Autodesk Inventor part; units mm, degrees
ref_plane "YZ Plane" through (0, 0, 0) normal (1, 0, 0) x (0, 1, 0)
ref_plane "XZ Plane" through (0, 0, 0) normal (0, 1, 0) x (-1, 0, 0)
ref_plane "XY Plane" through (0, 0, 0) normal (0, 0, 1) x (1, 0, 0)
sketch "Sketch1" plane through (0, 0, 0) normal (0, 1, 0) x (-1, 0, 0)
  circle A0 centre (0, 0) radius 25
  dimension "d1" = 50
extrude "Extrusion1" add sketch "Sketch1" along normal blind 12
sketch "Sketch2" plane through (0, 12, 0) normal (0, 1, 0) x (1, 0, 0)
  circle A0 centre (0, 0) radius 1.3723
  line L0 (-24.9867, -1.3423) -> (-24.9867, 1.3423) construction
  line L1 (-24.2459, -0.6015) -> (-24.2459, 0.6015)
  line L2 (-25.7274, 0.6015) -> (-25.7274, -0.6015)
  arc A1 (-25.7274, -0.6015) -> (-24.2459, -0.6015) centre (-24.9867, -0.6015) ccw
  arc A2 (-24.2459, 0.6015) -> (-25.7274, 0.6015) centre (-24.9867, 0.6015) ccw
  line L3 (1.3423, -24.9867) -> (-1.3423, -24.9867) construction
  line L4 (0.6015, -24.2459) -> (-0.6015, -24.2459)
  line L5 (-0.6015, -25.7274) -> (0.6015, -25.7274)
  arc A3 (0.6015, -25.7274) -> (0.6015, -24.2459) centre (0.6015, -24.9867) ccw
  arc A4 (-0.6015, -24.2459) -> (-0.6015, -25.7274) centre (-0.6015, -24.9867) ccw
  line L6 (24.9867, 1.3423) -> (24.9867, -1.3423) construction
  line L7 (24.2459, 0.6015) -> (24.2459, -0.6015)
  line L8 (25.7274, -0.6015) -> (25.7274, 0.6015)
  arc A5 (25.7274, 0.6015) -> (24.2459, 0.6015) centre (24.9867, 0.6015) ccw
  arc A6 (24.2459, -0.6015) -> (25.7274, -0.6015) centre (24.9867, -0.6015) ccw
  line L9 (-1.3423, 24.9867) -> (1.3423, 24.9867) construction
  line L10 (-0.6015, 24.2459) -> (0.6015, 24.2459)
  line L11 (0.6015, 25.7274) -> (-0.6015, 25.7274)
  arc A7 (-0.6015, 25.7274) -> (-0.6015, 24.2459) centre (-0.6015, 24.9867) ccw
  arc A8 (0.6015, 24.2459) -> (0.6015, 25.7274) centre (0.6015, 24.9867) ccw
  point P0 (-24.9867, 0)
  point P1 (0, -24.9867)
  point P2 (24.9867, 0)
  point P3 (0, 24.9867)
  dimension "d11" = 360
extrude "Extrusion2" cut sketch "Sketch2" against normal blind 12 contours A1 L2 A2 L1 | A3 L5 A4 L4 | A5 L8 A6 L7 | A7 L11 A8 L10
sketch "Sketch3" plane through (0, 12, 0) normal (0, 1, 0) x (1, 0, 0)
  circle A0 centre (0, 0) radius 22.8086
  arc A1 (13.2024, 18.5991) -> (2.9253, 22.6202) centre (0, 0) ccw construction
  arc A2 (13.9039, 19.5873) -> (3.0807, 23.822) centre (0, 0) ccw
  arc A3 (12.501, 17.611) -> (2.7699, 21.4184) centre (0, 0) ccw
  arc A4 (12.501, 17.611) -> (13.9039, 19.5873) centre (13.2024, 18.5991) ccw
  arc A5 (3.0807, 23.822) -> (2.7699, 21.4184) centre (2.9253, 22.6202) ccw
  line L0 (0, 0) -> (13.2024, 18.5991) construction
  line L1 (0, 0) -> (2.9253, 22.6202) construction
  arc A6 (-4.0188, 23.6818) -> (-14.6663, 19.0231) centre (0, 0) ccw
  arc A7 (-14.6663, 19.0231) -> (-13.1865, 17.1037) centre (-13.9264, 18.0634) ccw
  arc A8 (-3.6133, 21.2924) -> (-13.1865, 17.1037) centre (0, 0) ccw
  arc A9 (-3.6133, 21.2924) -> (-4.0188, 23.6818) centre (-3.816, 22.4871) ccw
  arc A10 (-19.5873, 13.9039) -> (-23.822, 3.0807) centre (0, 0) ccw
  arc A11 (-23.822, 3.0807) -> (-21.4184, 2.7699) centre (-22.6202, 2.9253) ccw
  arc A12 (-17.611, 12.501) -> (-21.4184, 2.7699) centre (0, 0) ccw
  arc A13 (-17.611, 12.501) -> (-19.5873, 13.9039) centre (-18.5991, 13.2024) ccw
  arc A14 (-23.6818, -4.0188) -> (-19.0231, -14.6663) centre (0, 0) ccw
  arc A15 (-19.0231, -14.6663) -> (-17.1037, -13.1865) centre (-18.0634, -13.9264) ccw
  arc A16 (-21.2924, -3.6133) -> (-17.1037, -13.1865) centre (0, 0) ccw
  arc A17 (-21.2924, -3.6133) -> (-23.6818, -4.0188) centre (-22.4871, -3.816) ccw
  arc A18 (-13.9039, -19.5873) -> (-3.0807, -23.822) centre (0, 0) ccw
  arc A19 (-3.0807, -23.822) -> (-2.7699, -21.4184) centre (-2.9253, -22.6202) ccw
  arc A20 (-12.501, -17.611) -> (-2.7699, -21.4184) centre (0, 0) ccw
  arc A21 (-12.501, -17.611) -> (-13.9039, -19.5873) centre (-13.2024, -18.5991) ccw
  arc A22 (4.0188, -23.6818) -> (14.6663, -19.0231) centre (0, 0) ccw
  arc A23 (14.6663, -19.0231) -> (13.1865, -17.1037) centre (13.9264, -18.0634) ccw
  arc A24 (3.6133, -21.2924) -> (13.1865, -17.1037) centre (0, 0) ccw
  arc A25 (3.6133, -21.2924) -> (4.0188, -23.6818) centre (3.816, -22.4871) ccw
  arc A26 (19.5873, -13.9039) -> (23.822, -3.0807) centre (0, 0) ccw
  arc A27 (23.822, -3.0807) -> (21.4184, -2.7699) centre (22.6202, -2.9253) ccw
  arc A28 (17.611, -12.501) -> (21.4184, -2.7699) centre (0, 0) ccw
  arc A29 (17.611, -12.501) -> (19.5873, -13.9039) centre (18.5991, -13.2024) ccw
  arc A30 (23.6818, 4.0188) -> (19.0231, 14.6663) centre (0, 0) ccw
  arc A31 (19.0231, 14.6663) -> (17.1037, 13.1865) centre (18.0634, 13.9264) ccw
  arc A32 (21.2924, 3.6133) -> (17.1037, 13.1865) centre (0, 0) ccw
  arc A33 (21.2924, 3.6133) -> (23.6818, 4.0188) centre (22.4871, 3.816) ccw
  dimension "d15" = 28
  dimension "d18" = 360
extrude "Extrusion3" cut sketch "Sketch3" against normal blind 12 contours A33 A32 A31 A0 | A0 A31 A30 A33 | A27 A26 A29 A0 | A0 A29 A28 A27 | A4 A3 A5 A0 | A0 A5 A2 A4 | A23 A22 A25 A0 | A0 A25 A24 A23 | A9 A8 A7 A0 | A0 A7 A6 A9 | A19 A18 A21 A0 | A0 A21 A20 A19 | A13 A12 A11 A0 | A0 A11 A10 A13 | A15 A14 A17 A0 | A0 A17 A16 A15
sketch "Sketch4" plane through (0, 12, 0) normal (0, 1, 0) x (1, 0, 0)
  circle A0 centre (0, 0) radius 4.43
  dimension "d22" = 8.86
extrude "Extrusion4" cut sketch "Sketch4" against normal blind 12
thread "Thread1"
sketch "Sketch5" plane through (0, 12, 0) normal (0, 1, 0) x (1, 0, 0)
  circle A0 centre (0, 0) radius 4.43
extrude "Extrusion5" [suppressed]
thread "Thread3"
thread "Thread4"
properties part number "ICRC wrist model"
Here's how the part is built. I have some questions about the finished solid (model axes, mm). A direction names the side the tool comes from. Coordinates: 2 decimals unless noted, no trailing zeros. Order: outer loops, then holes, each group sorted by start corner. A loop starts at its lowest first (then second) coordinate and runs counter-clockwise, first axis right, second up.
1) Imagine slicing it at C-C on z = -9. List the corners of the cut face in (x, y) for me, and give its area (3 significant figures).
2) I need wall thicknesses on line 1 (X direction, y = 6.75, z = 6); line 2 (Z direction, x = 18, y = 10); line 3 (Z direction, x = 5, y = 1.5). Which ranges of each line are inside material? Lowest first, please.
3) Imagine slicing it at B-B on x = 0. List the corners of the cut face in (y, z) for me, and give its area (3 significant figures).
4) We'd pull the mould along X, two halves only. Please class faces 1 (the face through (24.246, 6, 0)), 2 (the face through (22.04, 6.08, -9.55)): +X half, -X half, draft (parallel to the pull), parting line (faces both ways), or undercut.
5) Imagine slicing it at D-D on x = -7.5. List the corners of the cut face in (y, z) for me.
6) Imagine slicing it at A-A on z = 0. List the corners of the cut face in (x, y) for me.
7) Which directions (+Z, -Z, +X, -X, +Y, -Y) give clear straight access to the entire face, cutting with the end or side of a thin tool? Please do faces 3 (the face through (8.83, 6.08, -22.34)), 4 (the face through (17.496, 5.916, -17.858)).
8) Will these pins go through, and if not, where does the flat tip stop? pin 1 (4 mm diameter, centred on x = 5.5, y = 5, fed in from +Z); pin 2 (4 mm diameter, centred on y = 3.5, z = 18.5, fed in from +X); pin 3 (12 mm diameter, centred on x = -0.5, z = -3, fed in from -Y); pin 4 (1.3 mm diameter, centred on y = 8, z = 0, fed in from -X).
Response values:
1. outline: (-23.32, 0) - (-22.27, 0) - (-22.27, 12) - (-23.32, 12) - close; (-19.63, 0) - (19.63, 0) - (19.63, 12) - (-19.63, 12) - close; (22.27, 0) - (23.32, 0) - (23.32, 12) - (22.27, 12) - close
1. area: 496 mm2
2. line 1: x = -24.27 to -23.26, -20.75 to 20.75, 23.26 to 24.27
2. line 2: z = -17.35 to -15.14, -11.93 to 11.93, 14.26 to 17.35
2. line 3: z = -24.49 to -23.49, -21.01 to 21.01, 23.49 to 24.49
3. outline: (0, -24.25) - (12, -24.25) - (12, -4.43) - (0, -4.43) - close; (0, 4.43) - (12, 4.43) - (12, 24.25) - (0, 24.25) - close
3. area: 476 mm2
4. face 1: +X half
4. face 2: undercut
5. outline: (0, -23.85) - (12, -23.85) - (12, -22.82) - (0, -22.82) - close; (0, -20.25) - (12, -20.25) - (12, 20.25) - (0, 20.25) - close; (0, 22.82) - (12, 22.82) - (12, 23.85) - (0, 23.85) - close
6. outline: (-24.25, 0) - (-4.43, 0) - (-4.43, 12) - (-24.25, 12) - close; (4.43, 0) - (24.25, 0) - (24.25, 12) - (4.43, 12) - close
7. face 3: +Y, -Y
7. face 4: -Z, +X, +Y, -Y
8. pin 1: stops at z = 24.75
8. pin 2: stops at x = 18.78
8. pin 3: stops at y = 0
8. pin 4: stops at x = -24.25
